from build123d import *

# Parameters (mm, degrees)
BOSS_EXTRUDE1_DEPTH = 150
FILLET1_R           = 40
FILLET2_R           = 20
SKETCH7_R           = 80
CUT_EXTRUDE1_DEPTH  = 518.204021639


with BuildPart() as part:
    # Sketch2 → Boss-Extrude1 (new body)
    with BuildSketch(Plane.XY):
        Polygon((-75, 350), (75, 350), (75, 75), (350, 75), (350, -75), (75, -75), (75, -350), (-75, -350), (-75, -75), (-350, -75), (-350, 75), (-75, 75), align=None)
    extrude(amount=BOSS_EXTRUDE1_DEPTH)

    # Fillet1
    fillet1_edges = [part.edges().sort_by_distance(p)[0] for p in [
        (75, -350, 75),
        (-75, -350, 75),
        (-350, -75, 75),
        (-350, 75, 75),
        (-75, 350, 75),
        (75, 350, 75),
        (350, 75, 75),
        (350, -75, 75),
    ]]
    fillet(fillet1_edges, radius=FILLET1_R)

    # Fillet2
    fillet2_edges = [part.edges().sort_by_distance(p)[0] for p in [
        (-75, -192.5, 0),
        (-192.5, 75, 0),
        (75, 192.5, 0),
        (192.5, -75, 0),
        (0, 350, 0),
        (75, -192.5, 0),
        (0, -350, 0),
        (-192.5, -75, 0),
        (-350, 0, 0),
        (-75, 192.5, 0),
        (192.5, 75, 0),
        (350, 0, 0),
        (338.284271247, 63.284271247, 0),
        (338.284271247, -63.284271247, 0),
        (63.284271247, -338.284271247, 0),
        (-63.284271247, -338.284271247, 0),
        (-338.284271247, -63.284271247, 0),
        (-338.284271247, 63.284271247, 0),
        (-63.284271247, 338.284271247, 0),
        (63.284271247, 338.284271247, 0),
    ]]
    fillet(fillet2_edges, radius=FILLET2_R)

    # Sketch7 → Cut-Extrude1 (cut, through all)
    with BuildSketch(Plane.XY):
        with Locations(Location((0, 0, 0), (0, 0, 136.567463442))):
            Circle(SKETCH7_R)
    extrude(amount=CUT_EXTRUDE1_DEPTH, mode=Mode.SUBTRACT)


solid = part.part
Part model, mm, in its own coordinate system. A direction names the side the tool comes from. Give positions to 0.01 mm unless a question says otherwise; leave off trailing zeros. Order: outer loops, then holes, each group sorted by start corner. A loop starts at its lowest first (then second) coordinate and runs counter-clockwise, first axis right, second up. Notation, with made-up numbers: (20.5, -18) -> (59.5, -18) arc R15 cw to (59.5, 4) -> close; hole circle Ø5 at (9.25, 87.5). An arc over 180 degrees is marked (long way). Use one line per item in the form item = value.
(1) Saw through at D-D (y = 169.5). Write the cut outline in (x, z), then the cut area to 3 significant figures.
Solution:
outline = (-75, 20) arc R20 ccw to (-55, 0) -> (55, 0) arc R20 ccw to (75, 20) -> (75, 150) -> (-75, 150) -> close
area = 22,300 mm²
(2) Flat gauge pins, fed straight in: P1, Ø2, axis at x = -100.5, z = 127, coming from the +Y side; P2, Ø1.5, axis at y = -151, z = 48, coming from the +X side; P3, Ø2, axis at y = 261.5, z = 87, coming from the -X side. Where does each tip first touch, or does it go through?
Solution:
P1 = 75
P2 = 75
P3 = -75
(3) Saw through at C-C (z = 137.5). Write the cut outline in (x, y).
Solution:
outline = (-350, -35) arc R40 ccw to (-310, -75) -> (-75, -75) -> (-75, -310) arc R40 ccw to (-35, -350) -> (35, -350) arc R40 ccw to (75, -310) -> (75, -75) -> (310, -75) arc R40 ccw to (350, -35) -> (350, 35) arc R40 ccw to (310, 75) -> (75, 75) -> (75, 310) arc R40 ccw to (35, 350) -> (-35, 350) arc R40 ccw to (-75, 310) -> (-75, 75) -> (-310, 75) arc R40 ccw to (-350, 35) -> close; hole circle Ø160 at (0, 0)
(4) Saw through at A-A (y = 0). Write the cut outline in (x, z).
Solution:
outline = (-350, 20) arc R20 ccw to (-330, 0) -> (-80, 0) -> (-80, 150) -> (-350, 150) -> close; (80, 0) -> (330, 0) arc R20 ccw to (350, 20) -> (350, 150) -> (80, 150) -> close
(5) Tool access for faces 1 (the face through (75, -191, 84)), 2 (the face through (191, 75, 84)), 3 (the face through (-68.986, 185.058, 5.703)), 4 (the face through (-185.058, -68.986, 5.703)), 5 (the face through (181.51, -68.986, 5.703)): list every direction of +Z, -Z, +X, -X, +Y, -Y with a clear straight run to the whole face (end or side of a thin tool).
Solution:
face_1 = +Z, -Z, +X, -Y
face_2 = +Z, -Z, +X, +Y
face_3 = -Z, -X, +Y
face_4 = -Z, -X, -Y
face_5 = -Z, +X, -Y
(6) Drill centre lines: line 1 (X direction, y = 0, z = 95); line 2 (X direction, y = 99, z = 68). Where is each one in solid material? Low to high. Write a range as from..to.
Solution:
line_1 = -350..-80, 80..350
line_2 = -75..75
